The listing builds one solid part. Answer for the finished solid, in the listing's coordinates (mm). A direction names the side the tool comes from. Round coordinates to 2 decimals unless told otherwise and drop trailing zeros. Write each loop counter-clockwise with the first axis right and the second up, starting at its lowest first coordinate (ties: lowest second). Pieces come first, ordered by that corner, then holes. Notation, with made-up numbers: (0, 52.25) - (53, 52.25) arc R16 cw to (53, 60.25) - close; hole circle Ø6 at (42.5, 10). An arc over 180 degrees is marked (long way). Answer in a Markdown table with one row per item.
from build123d import *

# Parameters (mm, degrees)
F0_W     = 1400
F0_H     = 1308.4111795891
F1_DEPTH = 20
F2_DEPTH = 1385
F3_T     = -2.5


with BuildPart() as f1:
    # F0 (on Front) → F1 (new body)
    with BuildSketch(Plane.XZ):
        with Locations((-30.7828634977, 21.6243253089)):
            Rectangle(F0_W, F0_H)
    extrude(amount=F1_DEPTH)

    # F2 (add): faces of the model
    f2_faces = [f1.faces().sort_by_distance(p)[0] for p in [
        (-30.7828634977, -20, 21.6243253089),
        (-30.7828634977, 0, 21.6243253089),
    ]]
    extrude(f2_faces, amount=-F2_DEPTH, dir=(0, -1, 0))

    # F3
    f3_openings = [f1.faces().sort_by_distance(p)[0] for p in [
        (-30.782863, -20, 21.624325),
    ]]
    offset(amount=F3_T, openings=f3_openings)


solid = f1.part
(1) A flat-ended cylindrical pin translates along its axis: pin 1 (10 mm diameter, centred on x = -311, z = 160.5, fed in from -Y). Find the tip coordinate at first contact, or state that the pin passes through.
Checked values:
| item | result |
|---|---|
| pin 1 | stops at y = 1382.5 |
(2) Section C-C (x = 404) is taken. Give the vertices of the cut face in (y, z).
Checked values:
| item | result |
|---|---|
| outline | (-20, -632.58) - (1385, -632.58) - (1385, 675.83) - (-20, 675.83) - (-20, 673.33) - (1382.5, 673.33) - (1382.5, -630.08) - (-20, -630.08) - close |
(3) For faces 5 (the flat face through (-41, 671, 673.33)), 6 (the flat face through (-730.783, 673, 12)), determine the directions among +Z, -Z, +X, -X, +Y, -Y from which every point of the face is accessible in a straight line to the end or side of a thin tool.
Checked values:
| item | result |
|---|---|
| face 5 | -Y |
| face 6 | +Z, -Z, -X, +Y, -Y |
(4) Find the intervals of material crossed by line 1 (X direction, y = 879.5, z = 483.5); line 2 (Z direction, x = -72.5, y = 705); line 3 (Y direction, x = -177, z = 443.5), in increasing order.
Checked values:
| item | result |
|---|---|
| line 1 | x = -730.78 to -728.28, 666.72 to 669.22 |
| line 2 | z = -632.58 to -630.08, 673.33 to 675.83 |
| line 3 | y = 1382.5 to 1385 |
(5) For a pull along Z with two mould halves and no side action, classify faces 1 (the flat face through (-41, 673, 675.83)), 2 (the flat face through (669.217, 673, 12)), 3 (the flat face through (666.717, 671, 13)), 4 (the flat face through (-41, 673, -632.581)) as pulls with the +Z half, pulls with the -Z half, needs draft (parallel to the pull), parting line crosses it, or undercut.
Checked values:
| item | result |
|---|---|
| face 1 | pulls with the +Z half |
| face 2 | needs draft |
| face 3 | undercut |
| face 4 | pulls with the -Z half |
(6) Section B-B (z = 287) is taken. Give the vertices of the cut face in (x, y).
Checked values:
| item | result |
|---|---|
| outline | (-730.78, -20) - (-728.28, -20) - (-728.28, 1382.5) - (666.72, 1382.5) - (666.72, -20) - (669.22, -20) - (669.22, 1385) - (-730.78, 1385) - close |
(7) Section A-A (y = 651) is taken. Give the vertices of the cut face in (x, z).
Checked values:
| item | result |
|---|---|
| outline | (-730.78, -632.58) - (669.22, -632.58) - (669.22, 675.83) - (-730.78, 675.83) - close; hole (-728.28, -630.08) - (666.72, -630.08) - (666.72, 673.33) - (-728.28, 673.33) - close |
